from build123d import *

# Parameters (mm, degrees)
SKETCH_1_W          = 15
SKETCH_1_H          = 65
EXTRUDE_1_DEPTH     = 3
SKETCH_2_R          = 3
SKETCH_2_W          = 15
SKETCH_2_H          = 25
CUT_EXTRUDE_1_DEPTH = 3
SKETCH_4_W          = 2
SKETCH_4_H          = 65
EXTRUDE_2_DEPTH     = 69
SKETCH_5_W          = 6
SKETCH_5_H          = 25
CUT_EXTRUDE_2_DEPTH = 69
SKETCH_6_R          = 1.25
CUT_EXTRUDE_3_DEPTH = 69


with BuildPart() as part:
    # Sketch 1 → Extrude 1 (new body)
    with BuildSketch(Plane.XY):
        with Locations((7.5, 32.5)):
            Rectangle(SKETCH_1_W, SKETCH_1_H)
    extrude(amount=EXTRUDE_1_DEPTH)

    # Sketch 2 → Cut-Extrude 1 (cut)
    with BuildSketch(Plane.XY.offset(3)):
        with Locations((10, 57.5)):
            Circle(SKETCH_2_R)
        with Locations((10, 7.5)):
            Circle(SKETCH_2_R)
        with Locations((7.5, 32.5)):
            Rectangle(SKETCH_2_W, SKETCH_2_H)
    extrude(amount=-CUT_EXTRUDE_1_DEPTH, mode=Mode.SUBTRACT)


with BuildPart() as cut_extrude_1_piece_1:
    # of the separate pieces the step leaves, piece 1, a body of its own (cut_extrude_1_pieces)
    add(part.part.solids().sort_by_distance((0, 0, 0))[0])



with BuildPart() as cut_extrude_1_piece_2:
    # of the separate pieces the step leaves, piece 2, a body of its own (cut_extrude_1_pieces)
    add(part.part.solids().sort_by_distance((0, 65, 0))[0])


with BuildPart() as cut_extrude_1_piece_1_1:
    add(cut_extrude_1_piece_1.part)

    add(cut_extrude_1_piece_2.part)  # Extrude 2 merges Cut-Extrude 1 piece 2
    # Sketch 4 → Extrude 2 (add)
    with BuildSketch(Plane.XY.offset(3)):
        with Locations((1, 32.5)):
            Rectangle(SKETCH_4_W, SKETCH_4_H)
    extrude(amount=EXTRUDE_2_DEPTH)

    # Sketch 5 → Cut-Extrude 2 (cut)
    with BuildSketch(Plane(origin=(2, 0, 0), x_dir=(0, 0, -1), z_dir=(1, 0, 0))):
        with Locations((-6, 32.5)):
            Rectangle(SKETCH_5_W, SKETCH_5_H)
    extrude(amount=-CUT_EXTRUDE_2_DEPTH, mode=Mode.SUBTRACT)

    # Sketch 6 → Cut-Extrude 3 (cut)
    with BuildSketch(Plane(origin=(2, 0, 0), x_dir=(0, 0, -1), z_dir=(1, 0, 0))):
        with Locations(Location((-69.5, 62.5, 0), (0, 0, 90))):
            Circle(SKETCH_6_R)
        with Locations(Location((-10.5, 62.5, 0), (0, 0, 90))):
            Circle(SKETCH_6_R)
        with Locations(Location((-69.5, 2.5, 0), (0, 0, 90))):
            Circle(SKETCH_6_R)
        with Locations(Location((-10.5, 2.5, 0), (0, 0, 90))):
            Circle(SKETCH_6_R)
    extrude(amount=-CUT_EXTRUDE_3_DEPTH, mode=Mode.SUBTRACT)


solid = cut_extrude_1_piece_1_1.part
Geometry: final body of the model. Coordinates: model frame, mm. A direction names the side the tool comes from. Coordinates: 2 decimals unless noted, no trailing zeros. Order: outer loops, then holes, each group sorted by start corner. A loop starts at its lowest first (then second) coordinate and runs counter-clockwise, first axis right, second up.
(1) Access query for faces 4 (the face through (8, 10, 3)), 5 (the face through (1.01, 2.34, 70.74)), 6 (the face through (1, 32, 9)). Directions: +Z, -Z, +X, -X, +Y, -Y. A direction counts if a zero-diameter tool reaches every point of the face in a straight line with its end or side. Return the directions, or none.
(2) Draft query along Y for faces 1 (the face through (7, 55, 3)), 2 (the face through (12.77, 6.35, 1.52)), 3 (the face through (1, 0, 30)). Return one class per face: pulls with the +Y half, pulls with the -Y half, needs draft (parallel to the pull), parting line crosses it, or undercut.
(3) First-contact query: pin 1 (1 mm diameter, centred on x = 8, y = 15.5, fed in from +Z); pin 2 (0.6 mm diameter, centred on x = 1, y = 28.5, fed in from -Z); pin 3 (6 mm diameter, centred on y = 48.5, z = 50, fed in from +X). Flat tips, straight axial feed; report the tip coordinate or a pass-through.
(4) Section query B-B (z = 69.5). Return the cut outline in (x, y).
(5) Section query A-A (x = 10). Return the cut outline in (y, z).
(6) Material intervals for probe 1 along Y at (x, z) = (1.1, 69.5); probe 2 along Z at (x, y) = (1.55, 62.5); probe 3 along Z at (x, y) = (14.25, 7.5), sorted ascending.
(7) Section query D-D (x = 3.25). Return the cut outline in (y, z).
(8) Section query C-C (y = 62.5). Return the cut outline in (x, z).
Solution:
1. face 4: +Z, +X, +Y, -Y
1. face 5: +X, -X
1. face 6: -Z, +X, -X
2. face 1: needs draft
2. face 2: undercut
2. face 3: pulls with the -Y half
3. pin 1: stops at z = 3
3. pin 2: stops at z = 9
3. pin 3: stops at x = 2
4. outline: (0, 0) - (2, 0) - (2, 1.25) - (0, 1.25) - close; (0, 3.75) - (2, 3.75) - (2, 61.25) - (0, 61.25) - close; (0, 63.75) - (2, 63.75) - (2, 65) - (0, 65) - close
5. outline: (0, 0) - (4.5, 0) - (4.5, 3) - (0, 3) - close; (10.5, 0) - (20, 0) - (20, 3) - (10.5, 3) - close; (45, 0) - (54.5, 0) - (54.5, 3) - (45, 3) - close; (60.5, 0) - (65, 0) - (65, 3) - (60.5, 3) - close
6. probe 1: y = 0 to 1.25, 3.75 to 61.25, 63.75 to 65
6. probe 2: z = 0 to 9.25, 11.75 to 68.25, 70.75 to 72
6. probe 3: z = 0 to 3
7. outline: (0, 0) - (20, 0) - (20, 3) - (0, 3) - close; (45, 0) - (65, 0) - (65, 3) - (45, 3) - close
8. outline: (0, 0) - (15, 0) - (15, 3) - (2, 3) - (2, 9.25) - (0, 9.25) - close; (0, 11.75) - (2, 11.75) - (2, 68.25) - (0, 68.25) - close; (0, 70.75) - (2, 70.75) - (2, 72) - (0, 72) - close
